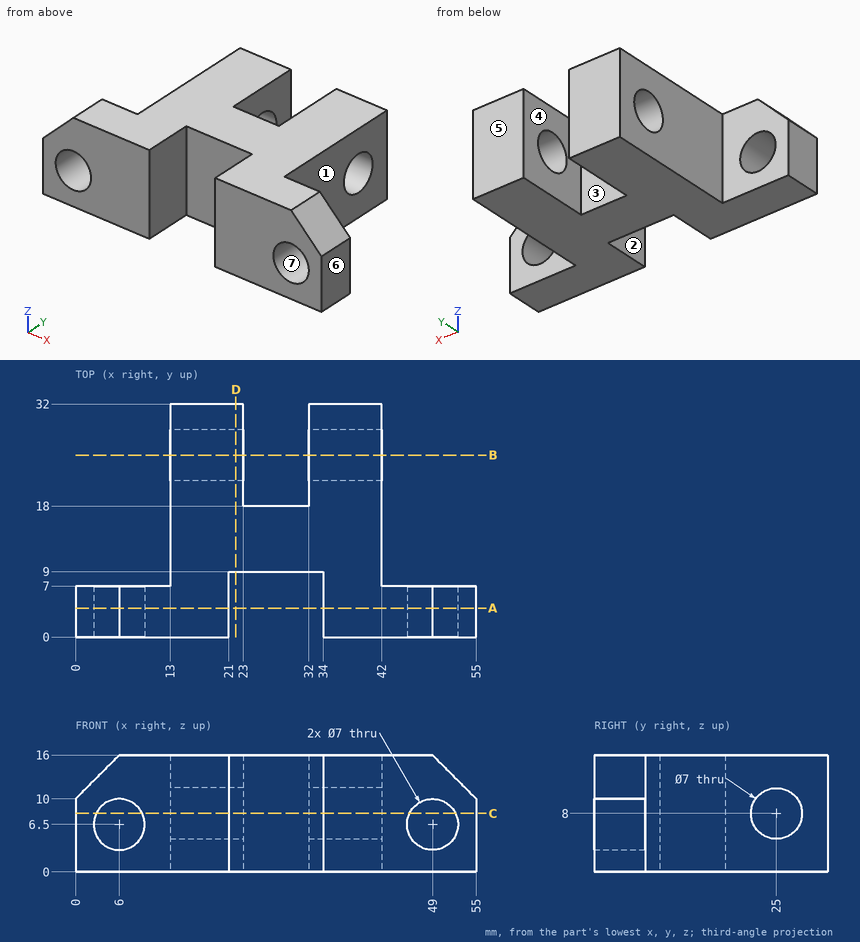
Study the drawing (mm; zero at the part's minimum x, y, z) and answer. A direction names the side the tool comes from. Coordinates: 2 decimals unless noted, no trailing zeros. Write each loop counter-clockwise with the first axis right and the second up, starting at its lowest first coordinate (ties: lowest second). Pieces come first, ordered by that corner, then holes.
Q1. Each of these flat-tipped pins is pushed along its axis until it touches: pin 1 Ø4.5 at (x, z) = (26, 7) entering from +Y; pin 2 Ø5 at (y, z) = (18, 7) entering from -X; pin 3 Ø6.5 at (x, z) = (45.5, 7) entering from +Y. Where does it stop, or does it pass through?
Q2. A cutting plane is placed at B-B, the plane y = 25. Give the vertices of the cut face in (x, z).
Q3. A cutting plane is placed at A-A, the plane y = 4. Give the vertices of the cut face in (x, z), then the cut area to 3 significant figures.
Q4. A cutting plane is placed at D-D, the plane x = 22. Give the vertices of the cut face in (y, z).
Q5. Find the intervals of material crossed by line 1 (X direction, y = 28.5, z = 2.5); line 2 (Z direction, x = 49, y = 5.75); line 3 (Z direction, x = 38, y = 25), in increasing order.
Q6. Which of the six approach directions +Z, -Z, +X, -X, +Y, -Y give full straight-line access (tool end or side, diameter ignored) to the marked faces 1, 2 and 3?
Q7. Determine the mould class of the marked faces 4, 5, 6 and 7 for opening direction X: released by +X, released by -X, zero draft, split by the parting line, or undercut.
Q8. A cutting plane is placed at C-C, the plane z = 8. State how many separate pieces and enclosed holes the cut face has, then the cut area to 3 significant figures.
Findings below:
1. pin 1: stops at y = 18
1. pin 2: stops at x = 13
1. pin 3: stops at y = 7
2. outline: (13, 0) - (23, 0) - (23, 4.5) - (13, 4.5) - close; (13, 11.5) - (23, 11.5) - (23, 16) - (13, 16) - close; (32, 0) - (42, 0) - (42, 4.5) - (32, 4.5) - close; (32, 11.5) - (42, 11.5) - (42, 16) - (32, 16) - close
3. outline: (0, 0) - (21, 0) - (21, 16) - (6, 16) - (0, 10) - close; (34, 0) - (55, 0) - (55, 10) - (49, 16) - (34, 16) - close; hole circle Ø7 at (6, 6.5); hole circle Ø7 at (49, 6.5)
3. area: 559 mm2
4. outline: (9, 0) - (32, 0) - (32, 16) - (9, 16) - close; hole circle Ø7 at (25, 8)
5. line 1: x = 13 to 23, 32 to 42
5. line 2: z = 0 to 3, 10 to 16
5. line 3: z = 0 to 4.5, 11.5 to 16
6. face 1: +Z, -Z, +X, +Y
6. face 2: +Z, -Z, -Y
6. face 3: +Z, -Z, +Y
7. face 4: undercut
7. face 5: zero draft
7. face 6: released by +X
7. face 7: undercut
8. separate pieces: 5
8. enclosed holes: 0
8. area: 638 mm2
